Autodesk Inventor part; units mm, degrees
ref_plane "YZ Plane" through (0, 0, 0) normal (1, 0, 0) x (0, 1, 0)
ref_plane "XZ Plane" through (0, 0, 0) normal (0, 1, 0) x (-1, 0, 0)
ref_plane "XY Plane" through (0, 0, 0) normal (0, 0, 1) x (1, 0, 0)
sketch "Sketch1" plane through (0, 0, 0) normal (0, 1, 0) x (-1, 0, 0)
  line L0 (0, 0) -> (84, 0)
  line L1 (84, 0) -> (84, -84)
  line L2 (84, -84) -> (0, -84)
  line L3 (0, -84) -> (0, 0)
  line L4 (16, -16) -> (68, -16)
  line L5 (68, -16) -> (68, -68)
  line L6 (68, -68) -> (16, -68)
  line L7 (16, -68) -> (16, -16)
  line L8 (0, 0) -> (84, -84) construction
  line L9 (84, 0) -> (0, -84) construction
  line L10 (46, 0) -> (46, -16)
  line L11 (38, 0) -> (38, -16)
  line L12 (38, -68) -> (38, -84)
  line L13 (46, -68) -> (46, -84)
  line L14 (46, -76) -> (38, -76) construction
  line L15 (42, -76) -> (42, -68) construction
  line L16 (50, -16) -> (50, -68)
  line L17 (34, -68) -> (34, -16)
  dimension "d0" = 52
  dimension "d1" = 84
  dimension "d2" = 4
  dimension "d3" = 4
  dimension "d4" = 4
extrude "Extrusion1" add sketch "Sketch1" along normal blind 10 contours L0 L11 L4 L7 L6 L12 L2 L3 | L0 L1 L2 L13 L6 L5 L4 L10 | L17 L6 L7 L4 | L4 L5 L6 L16
extrude "Extrusion2" add sketch "Sketch1" along normal blind 5 contours L0 L10 L4 L11 | L4 L16 L6 L17 | L12 L6 L13 L2
extrude "Extrusion3" add sketch "Sketch1" against normal blind 10 contours L4 L16 L6 L17 | L17 L6 L7 L4 | L4 L5 L6 L16
fillet "Fillet1" radius 2 4 edges at (-68, -10, -42) (-42, -10, -16) (-16, -10, -42) (-42, -10, -68)
fillet "Fillet2" radius 3 2 edges at (-42, 5, 0) (-42, 5, -84)
equation "\"d0\" = inner_carriage_length - 2 * inner_carriage_width"
equation "\"d1\" = long_centerlegg_width"
equation "\"d2\" = cabel_shaft_size"
equation "\"d3\" = cabel_shaft_size"
equation "\"d4\" = cabel_shaft_size"
equation "\"d5\" = 0.5 * centerlegg_topplate_thicknes"
equation "\"d7\" = 0.5 * centerlegg_topplate_thicknes - centerlegg_grove_depth"
equation "\"d9\" = 0.5 * centerlegg_topplate_thicknes"
equation "\"centerlegg_topplate_thicknes\" = 20"
equation "\"centerlegg_grove_depth\" = 5"
properties part number "09_centerlegg_topplate"
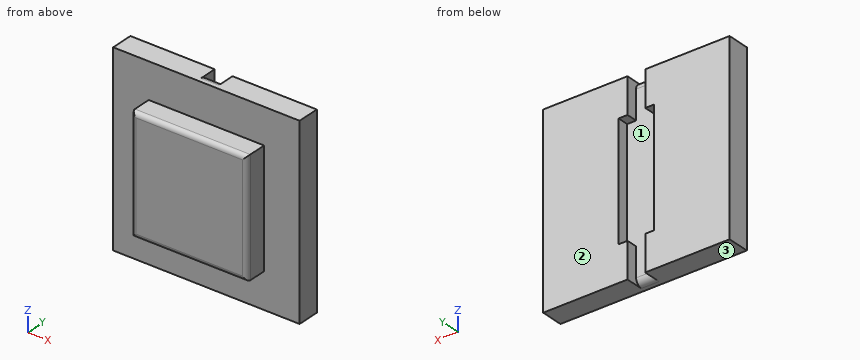
CAD build for the part. Positions are in the model's coordinates, mm. Face numbers are marked on the shaded views. Round coordinates to 2 decimals unless told otherwise and drop trailing zeros. Loops run counter-clockwise (first coordinate to the right, second up) from the corner with the lowest first, then second, coordinate; pieces in that order, holes last. Notation, with made-up numbers: M -31,26 L -7,26 A32 cw -7,54 Z; hole C 69.25,-9 d9. An arc over 180 degrees is marked long. Use a Markdown table: item, result. Add a question column.
(1) Cut at B-B (x = -39.5). Give the cut face in (y, z), and give its area (3 significant figures).
(2) Pull direction Z, two halves, no side cores. Call the marked faces 1, 2 and 3: +Z half, -Z half, draft (parallel to the pull), parting line (faces both ways), or undercut.
(3) Cut at D-D (z = -32). Give the cut face in (x, y), and give its area (3 significant figures).
(4) Drill centre lines: line 1 (X direction, y = 9, z = -44); line 2 (X direction, y = 8.75, z = -8); line 3 (Y direction, x = -14, z = -37.5). Where is each one in solid material? Low to high.
(5) Flat gauge pins, fed straight in: pin 1 (2 mm diameter, centred on x = -32.5, y = -2.5, fed in from +Z); pin 2 (6 mm diameter, centred on x = -62, y = -5, fed in from -Z); pin 3 (1.5 mm diameter, centred on y = -2.5, z = -33.5, fed in from -X). Where does each tip first touch, or does it go through?
(6) Cut at C-C (z = -72). Give the cut face in (x, y), and give its area (3 significant figures).
(7) Cut at A-A (y = 7). Give the cut face in (x, z), and give its area (3 significant figures).
Geometry says:
| question | item | result |
|---|---|---|
| 1 | outline | M -10,-66 A2 ccw -8,-68 L 0,-68 L 0,-84 L 2,-84 A3 ccw 5,-81 L 5,-3 A3 ccw 2,0 L 0,0 L 0,-16 L -8,-16 A2 ccw -10,-18 Z |
| 1 | area | 934 mm² |
| 2 | face 1 | undercut |
| 2 | face 2 | draft |
| 2 | face 3 | -Z half |
| 3 | outline | M -84,0 L -68,0 L -68,-8 A2 ccw -66,-10 L -18,-10 A2 ccw -16,-8 L -16,0 L 0,0 L 0,10 L -34,10 L -34,5 L -50,5 L -50,10 L -84,10 Z |
| 3 | area | 1,280 mm² |
| 4 | line 1 | x = -84 to -50, -34 to 0 |
| 4 | line 2 | x = -84 to -46, -38 to 0 |
| 4 | line 3 | y = 0 to 10 |
| 5 | pin 1 | stops at z = -16 |
| 5 | pin 2 | stops at z = -68 |
| 5 | pin 3 | stops at x = -68 |
| 6 | outline | M -84,0 L 0,0 L 0,10 L -38,10 L -38,5 L -46,5 L -46,10 L -84,10 Z |
| 6 | area | 800 mm² |
| 7 | outline | M -84,-84 L -46,-84 L -46,-68 L -50,-68 L -50,-16 L -46,-16 L -46,0 L -84,0 Z; M -38,-84 L 0,-84 L 0,0 L -38,0 L -38,-16 L -34,-16 L -34,-68 L -38,-68 Z |
| 7 | area | 5,970 mm² |
